```python
from build123d import *

# Parameters (mm, degrees)
F2_SIZE = 0.5


with BuildPart() as f1:
    # F0 (on Front) → F1 (revolve)
    with BuildSketch(Plane.XZ):
        with BuildLine():
            Line((5.131281, 75), (0, 75))
            Line((0, 75), (-5.131281, 75))
            Line((-5.131281, 75), (-5.131281, 72.5))
            Line((-5.131281, 72.5), (-10.131281, 72.5))
            Line((-10.131281, 72.5), (-10.131281, 75))
            Line((-10.131281, 75), (-15.131281, 75))
            Line((-15.131281, 75), (-15.131281, 72.5))
            Line((-15.131281, 72.5), (-20.131281, 72.5))
            Line((-20.131281, 72.5), (-20.131281, 75))
            Line((-20.131281, 75), (-25, 75))
            Line((-25, 75), (-25, 68.159989))
            Line((-25, 68.159989), (-17.565782, 63.867841))
            ThreePointArc((-17.565782, 63.867841), (-15.735655, 62.037714), (-15.065782, 59.537714))
            Line((-15.065782, 59.537714), (-15.065782, 42.5))
            ThreePointArc((-15.065782, 42.5), (-16.530248, 38.964466), (-20.065782, 37.5))
            Line((-20.065782, 37.5), (-25, 37.5))
            Line((-25, 37.5), (-25, 22.5))
            Line((-25, 22.5), (-20, 22.5))
            Line((-20, 22.5), (-20, 27.5))
            Line((-20, 27.5), (-15, 27.5))
            Line((-15, 27.5), (-15, 22.5))
            Line((-15, 22.5), (0, 22.5))
            Line((0, 22.5), (15, 22.5))
            Line((15, 22.5), (15, 27.5))
            Line((15, 27.5), (20, 27.5))
            Line((20, 27.5), (20, 22.5))
            Line((20, 22.5), (25, 22.5))
            Line((25, 22.5), (25, 37.5))
            Line((25, 37.5), (20.065782, 37.5))
            ThreePointArc((20.065782, 37.5), (16.530248, 38.964466), (15.065782, 42.5))
            Line((15.065782, 42.5), (15.065782, 59.537714))
            ThreePointArc((15.065782, 59.537714), (15.735655, 62.037714), (17.565782, 63.867841))
            Line((17.565782, 63.867841), (25, 68.159989))
            Line((25, 68.159989), (25, 75))
            Line((25, 75), (20.131281, 75))
            Line((20.131281, 75), (20.131281, 72.5))
            Line((20.131281, 72.5), (15.131281, 72.5))
            Line((15.131281, 72.5), (15.131281, 75))
            Line((15.131281, 75), (10.131281, 75))
            Line((10.131281, 75), (10.131281, 72.5))
            Line((10.131281, 72.5), (5.131281, 72.5))
            Line((5.131281, 72.5), (5.131281, 75))
        make_face()
    revolve(axis=Axis((-58.325773, 0, 0), (-1, 0, 0)))

    # F2
    f2_edges = [f1.edges().sort_by_distance(p)[0] for p in [
        (-15, 0, -22.5),
        (20, 0, -22.5),
        (15, 0, -22.5),
        (-20, 0, -22.5),
        (-25, 0, -22.5),
        (25, 0, -22.5),
        (15.131281, 0, -75),
        (5.131281, 0, -75),
        (-10.131281, 0, -75),
        (-20.131281, 0, -75),
        (-15.131281, 0, -75),
        (-5.131281, 0, -75),
        (10.131281, 0, -75),
        (20.131281, 0, -75),
    ]]
    chamfer(f2_edges, length=F2_SIZE)


solid = f1.part
```
Could you check a few things on this model? Use its own coordinates, in mm. A direction names the side the tool comes from. Round coordinates to 2 decimals unless told otherwise and drop trailing zeros. Loops run counter-clockwise (first coordinate to the right, second up) from the corner with the lowest first, then second, coordinate; pieces in that order, holes last. Notation, with made-up numbers: (37, -21.5) -> (84, -21.5) arc R21 cw to (84, -9.5) -> close; hole circle Ø3 at (-8, -34.5). An arc over 180 degrees is marked (long way). Put each result on its own line as item: value.
Q1. For pin 1 Ø12 at (x, z) = (20, 21.5) entering from -Y; pin 2 Ø10 at (x, y) = (-8.5, -31) entering from -Z; pin 3 Ø1 at (x, y) = (7.5, -42.5) entering from -Z, each with a flat end and sliding along its axis, tell me the tip position at first contact or that it passes through.
Checks:
pin 1: y = -73.37
pin 2: z = -70.17
pin 3: z = -59.1
Q2. Please list where these lines run through material, in increasing order: line 1 (Y direction, x = 7.75, z = 0); line 2 (X direction, y = 25, z = -49.5); line 3 (X direction, y = -59, z = 28.5). Write a range as from..to.
Checks:
line 1: -72.5..-22.5, 22.5..72.5
line 2: -15.07..15.07
line 3: -20.43..20.43
Q3. Thinking about a two-plate mould opening in X: for faces 4 (the cylindrical face through (-22.846, 74.362, -9.764)), 5 (the flat face through (15, -18.2, 14.4)), 6 (the flat face through (-15.066, 14, -41)), 7 (the conical face through (18.03, 43.35, -47.27)), which applies, pulls with the +X half, pulls with the -X half, needs draft (parallel to the pull), parting line crosses it, or undercut?
Checks:
face 4: needs draft
face 5: undercut
face 6: pulls with the -X half
face 7: pulls with the +X half
Q4. Which directions (+Z, -Z, +X, -X, +Y, -Y) give clear straight access to the entire face, cutting with the end or side of a thin tool? Please do faces 1 (the cylindrical face through (7.6, 21.78, 69.15)), 2 (the cylindrical face through (22.528, -19.961, 10.382)), 3 (the flat face through (15.066, 14, 41)).
Checks:
face 1: none
face 2: +X, -X
face 3: +X
Q5. I want a section at A-A on x = -7.5. Write out the boundary of the cut face in (y, z), and give its area (3 significant figures).
Checks:
outline: circle Ø145 at (0, 0); hole circle Ø45 at (0, 0)
area: 14,900 mm2
